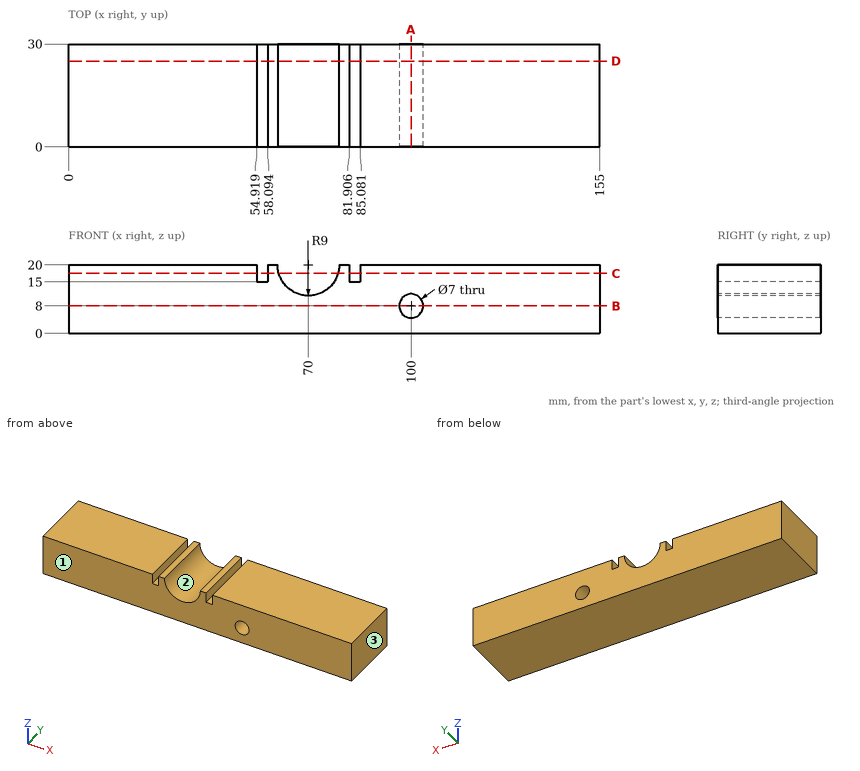
For this review, use the dimensioned drawing (mm, ordinates from the lowest corner) and the shaded views. Coordinates: 2 decimals unless noted, no trailing zeros. Loops run counter-clockwise (first coordinate to the right, second up) from the corner with the lowest first, then second, coordinate; pieces in that order, holes last. Notation, with made-up numbers: (62, 55) -> (107, 55) arc R25 ccw to (107, 70) -> close; hole circle Ø11 at (2.25, -38.5). An arc over 180 degrees is marked (long way). Use a Markdown table: item, result. Add a question column.
1. To check wall thickness, follow line 1 (X direction, y = 19.5, z = 19.25); line 2 (X direction, y = 20.25, z = 18.75); line 3 (Z direction, x = 100, y = 16). State the ranges of each line that lie inside material, in increasing order.
2. Add section C-C on z = 17.5. Write out the cut boundary in (x, y), plus the area to 3 significant figures.
3. Draft analysis for pull direction X (two halves, no side actions). For the marked faces 1, 2 and 3, state which applies: pulls with the +X half, pulls with the -X half, needs draft (parallel to the pull), parting line crosses it, or undercut.
4. Add section A-A on x = 100. Write out the cut boundary in (y, z), plus the area to 3 significant figures.
5. Add section D-D on y = 25. Write out the cut boundary in (x, z).
6. Clearance check with a flat-ended pin moving along its axis: pin 1 Ø1.6 at (x, y) = (83.5, 17.5) entering from +Z. State where the tip first meets the part, or that it passes through.
7. Add section B-B on z = 8. Write out the cut boundary in (x, y), plus the area to 3 significant figures.
Returned:
| question | item | result |
|---|---|---|
| 1 | line 1 | x = 0 to 54.92, 58.09 to 61.03, 78.97 to 81.91, 85.08 to 155 |
| 1 | line 2 | x = 0 to 54.92, 58.09 to 61.09, 78.91 to 81.91, 85.08 to 155 |
| 1 | line 3 | z = 0 to 4.5, 11.5 to 20 |
| 2 | outline | (0, 0) -> (54.92, 0) -> (54.92, 30) -> (0, 30) -> close; (58.09, 0) -> (61.35, 0) -> (61.35, 30) -> (58.09, 30) -> close; (78.65, 0) -> (81.91, 0) -> (81.91, 30) -> (78.65, 30) -> close; (85.08, 0) -> (155, 0) -> (155, 30) -> (85.08, 30) -> close |
| 2 | area | 3,940 mm² |
| 3 | face 1 | needs draft |
| 3 | face 2 | undercut |
| 3 | face 3 | pulls with the +X half |
| 4 | outline | (0, 0) -> (30, 0) -> (30, 4.5) -> (0, 4.5) -> close; (0, 11.5) -> (30, 11.5) -> (30, 20) -> (0, 20) -> close |
| 4 | area | 390 mm² |
| 5 | outline | (0, 0) -> (155, 0) -> (155, 20) -> (85.08, 20) -> (85.08, 15) -> (81.91, 15) -> (81.91, 20) -> (79, 20) arc R9 cw to (61, 20) -> (58.09, 20) -> (58.09, 15) -> (54.92, 15) -> (54.92, 20) -> (0, 20) -> close; hole circle Ø7 at (100, 8) |
| 6 | pin 1 | stops at z = 15 |
| 7 | outline | (0, 0) -> (96.5, 0) -> (96.5, 30) -> (0, 30) -> close; (103.5, 0) -> (155, 0) -> (155, 30) -> (103.5, 30) -> close |
| 7 | area | 4,440 mm² |
